Design review of the part built by this model. Coordinates are the model's own, in mm. Face numbers are marked on the shaded views. A direction names the side the tool comes from. Coordinates: 2 decimals unless noted, no trailing zeros. Loops run counter-clockwise (first coordinate to the right, second up) from the corner with the lowest first, then second, coordinate; pieces in that order, holes last. Notation, with made-up numbers: (66.25, 61.25) -> (87.25, 61.25) arc R30 cw to (87.25, 89.25) -> close; hole circle Ø1 at (-11.5, 3). An arc over 180 degrees is marked (long way). One line per item, written item: value. Start each with the question number.
1. Add section D-D on z = 5.5. Write out the cut boundary in (x, y), plus the area to 3 significant figures.
2. Add section A-A on x = 4. Write out the cut boundary in (y, z), plus the area to 3 significant figures.
3. Machinability: for the marked faces 4, 5 and 6, which of the approach directions +Z, -Z, +X, -X, +Y, -Y give a long, thin tool a straight path to every point of the face, cutting with its end or side? Answer none if there is none.
4. Insertion check: pin 1 (4.5 mm diameter, centred on x = 6.5, z = 12.5, fed in from -Y); pin 2 (7 mm diameter, centred on x = 4, y = -11, fed in from +Z); pin 3 (6 mm diameter, centred on y = -8.5, z = 25, fed in from +X); pin 4 (3 mm diameter, centred on x = 23, y = -11, fed in from -Z). Each pin has a flat end and moves straight along its axis. Give the tip position at first contact, or say it passes through.
5. For probe 1 along Y at (x, z) = (23, -0.2); probe 2 along X at (y, z) = (-5.75, 11.5); probe 3 along Y at (x, z) = (4.5, 30), list the stretches that pass through material, from the lowest coordinate up.
6. Draft analysis for pull direction Y (two halves, no side actions). For the marked faces 1, 2 and 3, state which applies: pulls with the +Y half, pulls with the -Y half, needs draft (parallel to the pull), parting line crosses it, or undercut.
7. Add section C-C on y = -7.5. Write out the cut boundary in (x, z), plus the area to 3 significant figures.
8. Add section B-B on y = -11. Write out the cut boundary in (x, z), plus the area to 3 significant figures.
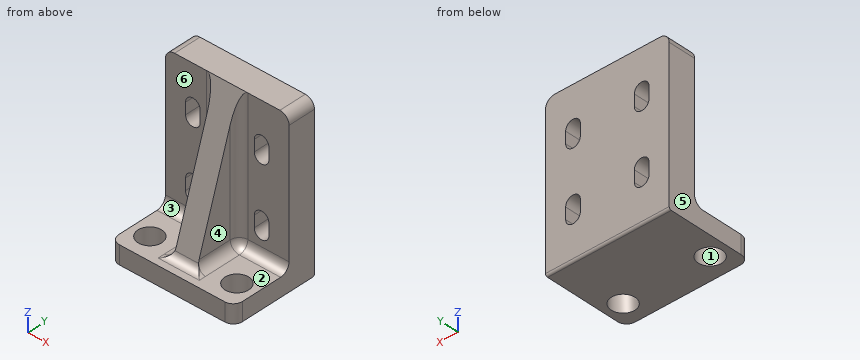
```python
from build123d import *

# Parameters (mm, degrees)
EXTRUDE_2_DEPTH      = 3
EXTRUDE_2_DEPTH_BACK = 1
SKETCH_1_W           = 27
SKETCH_1_H           = 16
EXTRUDE_4_DEPTH      = 3
EXTRUDE_4_DEPTH_BACK = 3
SKETCH_3_W           = 27
SKETCH_3_H           = 34
CUT_EXTRUDE_11_DEPTH = 13
EXTRUDE_5_DEPTH      = 2.5
EXTRUDE_5_DEPTH_BACK = 2.5
FILLET_2_R           = 2
FILLET_3_R           = 2
SKETCH_14_W          = 27
SKETCH_14_H          = 3
EXTRUDE_6_DEPTH      = 1
FILLET_5_R           = 0.5
SKETCH_16_R          = 2.6
CUT_EXTRUDE_12_DEPTH = 4


with BuildPart() as part:
    # 草图1 → 凸台-拉伸2 (new, two sides: drawn at the far end of the back side and taken through both)
    with BuildSketch(Plane.XY.offset(-EXTRUDE_2_DEPTH_BACK)):
        with Locations((13.5, -8)):
            Rectangle(SKETCH_1_W, SKETCH_1_H)
    extrude(amount=EXTRUDE_2_DEPTH + EXTRUDE_2_DEPTH_BACK)

    # 草图3 → 凸台-拉伸4 (add, two sides: drawn at the far end of the back side and taken through both)
    with BuildSketch(Plane(origin=(0, 0, 0), x_dir=(1, 0, 0), z_dir=(0, 1, 0)).offset(-EXTRUDE_4_DEPTH_BACK)):
        with Locations((13.5, -17)):
            Rectangle(SKETCH_3_W, SKETCH_3_H)
    extrude(amount=EXTRUDE_4_DEPTH + EXTRUDE_4_DEPTH_BACK)

    # 草图4 → 切除-拉伸11 (cut)
    with BuildSketch(Plane(origin=(0, -3, 0), x_dir=(-1, 0, 0), z_dir=(0, -1, 0))):
        with BuildLine():
            Line((-7.6, -10.5), (-7.6, -8))
            ThreePointArc((-7.6, -8), (-6, -6.4), (-4.4, -8))
            Line((-4.4, -8), (-4.4, -10.5))
            ThreePointArc((-4.4, -10.5), (-6, -12.1), (-7.6, -10.5))
        make_face()
        with BuildLine():
            Line((-22.6, -10.5), (-22.6, -8))
            ThreePointArc((-22.6, -8), (-21, -6.4), (-19.4, -8))
            Line((-19.4, -8), (-19.4, -10.5))
            ThreePointArc((-19.4, -10.5), (-21, -12.1), (-22.6, -10.5))
        make_face()
        with BuildLine():
            Line((-7.6, -25.5), (-7.6, -23))
            ThreePointArc((-7.6, -23), (-6, -21.4), (-4.4, -23))
            Line((-4.4, -23), (-4.4, -25.5))
            ThreePointArc((-4.4, -25.5), (-6, -27.1), (-7.6, -25.5))
        make_face()
        with BuildLine():
            Line((-22.6, -25.5), (-22.6, -23))
            ThreePointArc((-22.6, -23), (-21, -21.4), (-19.4, -23))
            Line((-19.4, -23), (-19.4, -25.5))
            ThreePointArc((-19.4, -25.5), (-21, -27.1), (-22.6, -25.5))
        make_face()
    extrude(amount=-CUT_EXTRUDE_11_DEPTH, mode=Mode.SUBTRACT)

    # 草图13 → 凸台-拉伸5 (add, two sides: drawn at the far end of the back side and taken through both)
    with BuildSketch(Plane.ZY.offset(-13.5).offset(-EXTRUDE_5_DEPTH_BACK)):
        Polygon((3, -13), (34, -3), (3, -3), align=None)
    extrude(amount=EXTRUDE_5_DEPTH + EXTRUDE_5_DEPTH_BACK)

    # 圆角2
    fillet_2_edges = [part.edges().sort_by_distance(p)[0] for p in [
        (21.5, -3, 3),
        (5.5, -3, 3),
        (0, 0, 34),
        (27, 0, 34),
        (0, -16, 1),
        (27, -16, 1),
    ]]
    fillet(fillet_2_edges, radius=FILLET_2_R)

    # 圆角3
    # the kernel refuses this fillet: 2 mm, written as the material it adds along each edge
    with BuildSketch(Plane(origin=(11, -13, 3), x_dir=(0, -1, 0), z_dir=(1, 0, 0))) as fillet_3_piece_1:
        with BuildLine():
            CenterArc((FILLET_3_R * 0.728161127413, -FILLET_3_R), FILLET_3_R, 90, 72.121303404)
            Line((-FILLET_3_R * 0.223547490347, -FILLET_3_R * 0.692997220077), (0, 0))
            Line((0, 0), (FILLET_3_R * 0.728161127413, 0))
        make_face()
    extrude(amount=5)
    with BuildSketch(Plane(origin=(16, -3, 34), x_dir=(0, -1, 0), z_dir=(0, 0, -1))) as fillet_3_piece_2_section:
        with BuildLine():
            CenterArc((FILLET_3_R, -FILLET_3_R), FILLET_3_R, 90, 90)
            Line((0, -FILLET_3_R), (0, 0))
            Line((0, 0), (FILLET_3_R, 0))
        make_face()
    fillet_3_piece_2 = extrude(amount=29, mode=Mode.PRIVATE)
    fillet_3_piece_2 = split(fillet_3_piece_2, bisect_by=Plane(origin=(16.465034927, -7.473683047, 20.131582554), z_dir=(0, 0.9517086177605509, -0.3070027799227584)), keep=Keep.TOP, mode=Mode.PRIVATE)
    add(fillet_3_piece_2)
    with BuildSketch(Plane(origin=(11, -3, 34), x_dir=(-1, 0, 0), z_dir=(0, 0, -1))) as fillet_3_piece_3_section:
        with BuildLine():
            CenterArc((FILLET_3_R, -FILLET_3_R), FILLET_3_R, 90, 90)
            Line((0, -FILLET_3_R), (0, 0))
            Line((0, 0), (FILLET_3_R, 0))
        make_face()
    fillet_3_piece_3 = extrude(amount=29, mode=Mode.PRIVATE)
    fillet_3_piece_3 = split(fillet_3_piece_3, bisect_by=Plane(origin=(10.534965073, -7.473683047, 20.131582554), z_dir=(0, 0.9517086177605509, -0.3070027799227584)), keep=Keep.TOP, mode=Mode.PRIVATE)
    add(fillet_3_piece_3)
    with BuildSketch(Plane(origin=(11, -5, 3), x_dir=(-1, 0, 0), z_dir=(0, -1, 0))) as fillet_3_piece_4_section:
        with BuildLine():
            CenterArc((FILLET_3_R, -FILLET_3_R), FILLET_3_R, 90, 90)
            Line((0, -FILLET_3_R), (0, 0))
            Line((0, 0), (FILLET_3_R, 0))
        make_face()
    fillet_3_piece_4 = extrude(amount=13, mode=Mode.PRIVATE)
    fillet_3_piece_4 = split(fillet_3_piece_4, bisect_by=Plane(origin=(10.542698912, -12.486166037, 4.592885286), z_dir=(0, 0.9517086177605509, -0.3070027799227584)), keep=Keep.TOP, mode=Mode.PRIVATE)
    add(fillet_3_piece_4)
    with BuildSketch(Plane(origin=(11, -5, 5), x_dir=(0, 0, -1), z_dir=(0, -1, 0))) as fillet_3_piece_5:
        with BuildLine():
            CenterArc((2 - FILLET_3_R, -FILLET_3_R), FILLET_3_R, 0, 90)
            Line((2 - FILLET_3_R, 0), (2, 0))
            Line((2, 0), (2, -FILLET_3_R))
        make_face()
    revolve(axis=Axis((11, -5, 5), (1, 0, 0)), revolution_arc=90)
    with BuildSketch(Plane(origin=(16, -5, 3), x_dir=(1, 0, 0), z_dir=(0, -1, 0))) as fillet_3_piece_6_section:
        with BuildLine():
            CenterArc((FILLET_3_R, FILLET_3_R), FILLET_3_R, 180, 90)
            Line((0, FILLET_3_R), (0, 0))
            Line((0, 0), (FILLET_3_R, 0))
        make_face()
    fillet_3_piece_6 = extrude(amount=13, mode=Mode.PRIVATE)
    fillet_3_piece_6 = split(fillet_3_piece_6, bisect_by=Plane(origin=(16.457301088, -12.486166037, 4.592885286), z_dir=(0, 0.9517086177605509, -0.3070027799227584)), keep=Keep.TOP, mode=Mode.PRIVATE)
    add(fillet_3_piece_6)
    with BuildSketch(Plane(origin=(16, -5, 5), x_dir=(0, 0, -1), z_dir=(0, -1, 0))) as fillet_3_piece_7:
        with BuildLine():
            CenterArc((2 - FILLET_3_R, FILLET_3_R), FILLET_3_R, 270, 90)
            Line((2 - FILLET_3_R, 0), (2, 0))
            Line((2, 0), (2, FILLET_3_R))
        make_face()
    revolve(axis=Axis((16, -5, 5), (1, 0, 0)), revolution_arc=90)
    with BuildSketch(Plane(origin=(11, -5, 3), x_dir=(-1, 0, 0), z_dir=(0, -1, 0))) as fillet_3_piece_8a_section:
        with BuildLine():
            CenterArc((FILLET_3_R, -FILLET_3_R), FILLET_3_R, 90, 90)
            Line((0, -FILLET_3_R), (0, 0))
            Line((0, 0), (FILLET_3_R, 0))
        make_face()
    fillet_3_piece_8a = extrude(amount=13, mode=Mode.PRIVATE)
    fillet_3_piece_8a = split(fillet_3_piece_8a, bisect_by=Plane(origin=(10.55847084, -16, 3.471852111), z_dir=(0, 1, 0)), keep=Keep.TOP, mode=Mode.PRIVATE)
    fillet_3_piece_8a = split(fillet_3_piece_8a, bisect_by=Plane(origin=(10.55847084, -12.996338669, 3.011350127), z_dir=(0, -0.9517086177605509, 0.3070027799227584)), keep=Keep.TOP, mode=Mode.PRIVATE)
    with BuildSketch(Plane(origin=(7.359194363, -13, 3), x_dir=(0, -1, 0), z_dir=(1, 0, 0))) as fillet_3_piece_8b_section:
        with BuildLine():
            CenterArc((FILLET_3_R * 0.728161127413, -FILLET_3_R), FILLET_3_R, 90, 72.121303404)
            Line((-FILLET_3_R * 0.223547490347, -FILLET_3_R * 0.692997220077), (0, 0))
            Line((0, 0), (FILLET_3_R * 0.728161127413, 0))
        make_face()
    fillet_3_piece_8b = extrude(amount=8.640805637, mode=Mode.PRIVATE)
    fillet_3_piece_8b = split(fillet_3_piece_8b, bisect_by=Plane(origin=(11, -13.221902521, 3.304743707), z_dir=(-1, 0, 0)), keep=Keep.TOP, mode=Mode.PRIVATE)
    fillet_3_piece_8 = fillet_3_piece_8a & fillet_3_piece_8b
    add(fillet_3_piece_8)
    with BuildSketch(Plane(origin=(16, -5, 3), x_dir=(1, 0, 0), z_dir=(0, -1, 0))) as fillet_3_piece_9a_section:
        with BuildLine():
            CenterArc((FILLET_3_R, FILLET_3_R), FILLET_3_R, 180, 90)
            Line((0, FILLET_3_R), (0, 0))
            Line((0, 0), (FILLET_3_R, 0))
        make_face()
    fillet_3_piece_9a = extrude(amount=13, mode=Mode.PRIVATE)
    fillet_3_piece_9a = split(fillet_3_piece_9a, bisect_by=Plane(origin=(16.44152916, -16, 3.471852111), z_dir=(0, 1, 0)), keep=Keep.TOP, mode=Mode.PRIVATE)
    fillet_3_piece_9a = split(fillet_3_piece_9a, bisect_by=Plane(origin=(16.44152916, -12.996338669, 3.011350127), z_dir=(0, -0.9517086177605509, 0.3070027799227584)), keep=Keep.TOP, mode=Mode.PRIVATE)
    with BuildSketch(Plane(origin=(11, -13, 3), x_dir=(0, -1, 0), z_dir=(1, 0, 0))) as fillet_3_piece_9b_section:
        with BuildLine():
            CenterArc((FILLET_3_R * 0.728161127413, -FILLET_3_R), FILLET_3_R, 90, 72.121303404)
            Line((-FILLET_3_R * 0.223547490347, -FILLET_3_R * 0.692997220077), (0, 0))
            Line((0, 0), (FILLET_3_R * 0.728161127413, 0))
        make_face()
    fillet_3_piece_9b = extrude(amount=8.640805637, mode=Mode.PRIVATE)
    fillet_3_piece_9b = split(fillet_3_piece_9b, bisect_by=Plane(origin=(16, -13.221902521, 3.304743707), z_dir=(1, 0, 0)), keep=Keep.TOP, mode=Mode.PRIVATE)
    fillet_3_piece_9 = fillet_3_piece_9a & fillet_3_piece_9b
    add(fillet_3_piece_9)

    # 草图14 → 凸台-拉伸6 (add)
    with BuildSketch(Plane(origin=(0, 0, 0), x_dir=(-1, 0, 0), z_dir=(0, 0, -1))):
        with Locations((-13.5, 1.5)):
            Rectangle(SKETCH_14_W, SKETCH_14_H)
    extrude(amount=EXTRUDE_6_DEPTH)

    # 圆角5
    fillet_5_edges = [part.edges().sort_by_distance(p)[0] for p in [
        (13.5, 3, -1),
    ]]
    fillet(fillet_5_edges, radius=FILLET_5_R)

    # 草图16 → 切除-拉伸12 (cut)
    with BuildSketch(Plane.XY.offset(3)):
        with Locations((4, -11)):
            Circle(SKETCH_16_R)
        with Locations((23, -11)):
            Circle(SKETCH_16_R)
    extrude(amount=-CUT_EXTRUDE_12_DEPTH, mode=Mode.SUBTRACT)


solid = part.part
```
Worked answers:
1. outline: (0, -3) -> (9, -3) arc R2 cw to (11, -5) -> (11, -12.19) -> (16, -12.19) -> (16, -5) arc R2 cw to (18, -3) -> (27, -3) -> (27, 3) -> (0, 3) -> close
1. area: 210 mm²
2. outline: (-16, -1) -> (-13.6, -1) -> (-13.6, 3) -> (-16, 3) -> close; (-8.4, -1) -> (2.5, -1) arc R0.5 ccw to (3, -0.5) -> (3, 34) -> (-3, 34) -> (-3, 5) arc R2 cw to (-5, 3) -> (-8.4, 3) -> close
2. area: 242 mm²
3. face 4: +Z, +X, -Y
3. face 5: +Z, -Z, -X, +Y, -Y
3. face 6: +Z, -X, -Y
4. pin 1: stops at y = -3
4. pin 2: stops at z = 3
4. pin 3: stops at x = 16
4. pin 4: passes through
5. probe 1: y = -16 to -13.6, -8.4 to 3
5. probe 2: x = 11 to 16
5. probe 3: y = -3 to 3
6. face 1: undercut
6. face 2: needs draft
6. face 3: pulls with the -Y half
7. outline: (0, -1) -> (27, -1) -> (27, 3) -> (18, 3) arc R2 cw to (16, 5) -> (16, 20.05) -> (11, 20.05) -> (11, 5) arc R2 cw to (9, 3) -> (0, 3) -> close
7. area: 195 mm²
8. outline: (0, -1) -> (1.4, -1) -> (1.4, 3) -> (0, 3) -> close; (6.6, -1) -> (20.4, -1) -> (20.4, 3) -> (18, 3) arc R2 cw to (16, 5) -> (16, 9.2) -> (11, 9.2) -> (11, 5) arc R2 cw to (9, 3) -> (6.6, 3) -> close; (25.6, -1) -> (27, -1) -> (27, 3) -> (25.6, 3) -> close
8. area: 99.1 mm²
